Verification items for the finished model (mm, model axes). Face numbers are marked on the shaded views. A direction names the side the tool comes from. Give positions to 0.01 mm unless a question says otherwise; leave off trailing zeros. Loops run counter-clockwise (first coordinate to the right, second up) from the corner with the lowest first, then second, coordinate; pieces in that order, holes last. Notation, with made-up numbers: (16, 32.5) - (49, 32.5) arc R25 cw to (49, 70.5) - close; hole circle Ø1 at (44.5, 78.5). An arc over 180 degrees is marked (long way). Put each result on its own line as item: value. Start each with the question number.
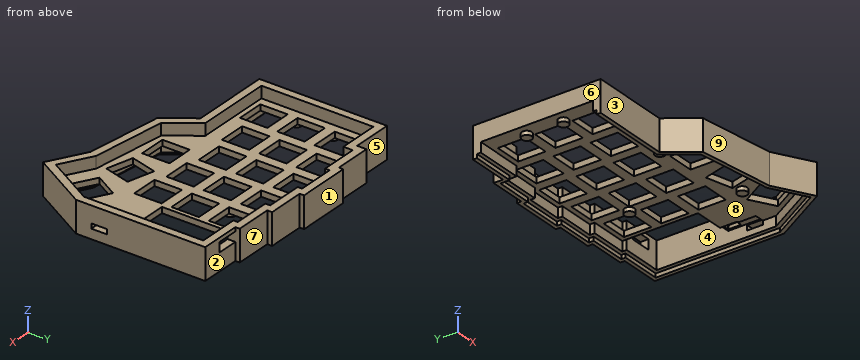
```python
from build123d import *

# Parameters (mm, degrees)
PAD005_DEPTH        = 16
POCKET_DEPTH        = 6
POCKET012_DEPTH     = 7
SKETCH001_W         = 14
SKETCH001_H         = 14
SKETCH001_W_2       = 20.75
SKETCH001_H_2       = 36.5
POCKET013_DEPTH     = 3
MIRROREDSKETCH009_R = 2.5
PAD_DEPTH           = 5
SKETCH_W            = 8
SKETCH_H            = 2.5
POCKET014_DEPTH     = 5
SKETCH015_W         = 11
SKETCH015_H         = 5
POCKET015_DEPTH     = 7
POCKET018_DEPTH     = 2
POCKET025_DEPTH     = 5
POCKET026_DEPTH     = 1.1


with BuildPart() as part:
    # MirroredSketch002 → Pad005 (new body)
    with BuildSketch(Plane.XY):
        Polygon((12.847899, 60.749919), (33.482443, 60.749919), (33.482443, 65.499919), (52.492443, 65.499919), (52.492443, 67.749919), (79.492443, 67.749919), (79.492443, 65.499919), (98.492443, 65.499919), (98.492443, 62.999919), (117.482443, 62.999919), (117.482443, 60.749919), (138.232443, 60.749919), (138.232443, -5.348885), (121.287497, -34.793261), (102.74032, -24.222717), (63.98748, -18.955575), (53.446293, -4.5), (12.847899, -4.5), align=None)
    extrude(amount=PAD005_DEPTH)

    # MirroredSketch005 → Pocket (cut)
    with BuildSketch(Plane.XY.offset(16)):
        Polygon((16.847899, -0.5), (16.847899, 56.75), (37.482443, 56.75), (37.482443, 61.499919), (56.492443, 61.499919), (56.492443, 63.749919), (75.492443, 63.749919), (75.492443, 61.499919), (94.492443, 61.499919), (94.492443, 58.999919), (113.482443, 58.999919), (113.482443, 56.749919), (134.232443, 56.749919), (134.232443, -4.280081), (119.807428, -29.345701), (104.047316, -20.363581), (66.215158, -15.221576), (55.48, -0.5), align=None)
    extrude(amount=-POCKET_DEPTH, mode=Mode.SUBTRACT)

    # MirroredSketch006 → Pocket012 (cut)
    with BuildSketch(Plane.XY):
        Polygon((-0.5, -0.5), (-0.5, 56.75), (37.482443, 56.75), (37.482443, 61.499919), (56.492443, 61.499919), (56.492443, 63.749919), (75.492443, 63.749919), (75.492443, 61.499919), (94.492443, 61.499919), (94.492443, 58.999919), (113.482443, 58.999919), (113.482443, 56.749919), (134.232443, 56.749919), (134.232443, -4.280081), (119.807428, -29.345701), (104.047316, -20.363581), (66.215158, -15.221576), (55.48, -0.5), align=None)
    extrude(amount=POCKET012_DEPTH, mode=Mode.SUBTRACT)

    # Sketch001 → Pocket013 (cut)
    with BuildSketch(Plane.XY.offset(10)):
        with Locations((75.62, -5.79)):
            Rectangle(SKETCH001_W, SKETCH001_H)
        Polygon((91.629303, 0.089303), (105.156052, -3.52), (101.546749, -17.046749), (88.02, -13.437445), align=None)
        Polygon((116.274632, -2.66), (128.398988, -9.66), (121.398988, -21.784355), (109.276749, -14.785577), align=None)
        with Locations((28.07, 47.16)):
            Rectangle(SKETCH001_W, SKETCH001_H)
        with Locations((28.07, 9.06)):
            Rectangle(SKETCH001_W, SKETCH001_H)
        with Locations((47.12, 51.97)):
            Rectangle(SKETCH001_W, SKETCH001_H)
        with Locations((47.12, 13.87)):
            Rectangle(SKETCH001_W, SKETCH001_H)
        with Locations((66.17, 54.27)):
            Rectangle(SKETCH001_W, SKETCH001_H)
        with Locations((66.17, 16.17)):
            Rectangle(SKETCH001_W, SKETCH001_H)
        with Locations((85.22, 51.87)):
            Rectangle(SKETCH001_W, SKETCH001_H)
        with Locations((85.22, 13.77)):
            Rectangle(SKETCH001_W, SKETCH001_H)
        with Locations((104.27, 49.54)):
            Rectangle(SKETCH001_W, SKETCH001_H)
        with Locations((47.12, 32.92)):
            Rectangle(SKETCH001_W, SKETCH001_H)
        with Locations((66.17, 35.22)):
            Rectangle(SKETCH001_W, SKETCH001_H)
        with Locations((28.07, 28.11)):
            Rectangle(SKETCH001_W, SKETCH001_H)
        with Locations((104.27, 30.49)):
            Rectangle(SKETCH001_W, SKETCH001_H)
        with Locations((104.27, 11.44)):
            Rectangle(SKETCH001_W, SKETCH001_H)
        with Locations((85.22, 32.82)):
            Rectangle(SKETCH001_W, SKETCH001_H)
        with Locations((123.857443, 38.499919)):
            Rectangle(SKETCH001_W_2, SKETCH001_H_2)
    extrude(amount=-POCKET013_DEPTH, mode=Mode.SUBTRACT)

    # MirroredSketch009 → Pad (join)
    with BuildSketch(Plane.XY.offset(10)):
        with Locations((18.61, 37.509997)):
            Circle(MIRROREDSKETCH009_R)
        with Locations((18.6, 18.76)):
            Circle(MIRROREDSKETCH009_R)
        with Locations((94.55, 41.252659)):
            Circle(MIRROREDSKETCH009_R)
        with Locations((61.84, 1.51)):
            Circle(MIRROREDSKETCH009_R)
        with Locations((108.3, -6.24)):
            Circle(MIRROREDSKETCH009_R)
    extrude(amount=-PAD_DEPTH)

    # Sketch → Pocket014 (cut)
    with BuildSketch(Plane.YZ.offset(138.3)):
        with Locations((6.479556, 6.26)):
            Rectangle(SKETCH_W, SKETCH_H)
    extrude(amount=-POCKET014_DEPTH, mode=Mode.SUBTRACT)

    # Sketch015 → Pocket015 (cut)
    with BuildSketch(Plane(origin=(6, 56.73, -16.55), x_dir=(1, 0, 0), z_dir=(0, -1, 0))):
        with Locations((116.982443, 28.05)):
            Rectangle(SKETCH015_W, SKETCH015_H)
    extrude(amount=-POCKET015_DEPTH, mode=Mode.SUBTRACT)

    # MirroredSketch013 → Pocket018 (cut)
    with BuildSketch(Plane.XY):
        Polygon((-2.5, 58.75), (35.482443, 58.75), (35.482443, 63.499919), (54.492443, 63.499919), (54.492443, 65.749919), (77.492443, 65.749919), (77.492443, 63.499919), (96.492443, 63.499919), (96.492443, 60.999919), (115.482443, 60.999919), (115.482443, 58.749919), (136.232443, 58.749919), (136.232443, -4.814483), (120.547462, -32.069481), (103.393818, -22.293149), (65.101319, -17.088576), (54.463147, -2.5), (-2.5, -2.5), align=None)
        Polygon((-0.5, -0.5), (-0.5, 56.75), (37.482443, 56.75), (37.482443, 61.499919), (56.492443, 61.499919), (56.492443, 63.749919), (75.492443, 63.749919), (75.492443, 61.499919), (94.492443, 61.499919), (94.492443, 58.999919), (113.482443, 58.999919), (113.482443, 56.749919), (134.232443, 56.749919), (134.232443, -4.280081), (119.807428, -29.345701), (104.047316, -20.363581), (66.215158, -15.221576), (55.48, -0.5), align=None, mode=Mode.SUBTRACT)
    extrude(amount=POCKET018_DEPTH, mode=Mode.SUBTRACT)

    # Sketch042 → Pocket025 (cut)
    with BuildSketch(Plane(origin=(131.5, 16.2, 8.1), x_dir=(1, 0, 0), z_dir=(0, 0, 1))):
        with BuildLine():
            ThreePointArc((-1.699662, -3.023679), (-1.602072, -3.215198), (-1.401398, -3.292227))
            Line((1.461956, -3.292227), (-1.401398, -3.292227))
            ThreePointArc((1.461956, -3.292227), (1.630798, -3.203454), (1.698398, -3.025076))
            Line((1.698398, 3.034671), (1.698398, -3.025076))
            ThreePointArc((1.698398, 3.034671), (1.611903, 3.194523), (1.444123, 3.264409))
            Line((-1.429415, 3.264409), (1.444123, 3.264409))
            ThreePointArc((-1.429415, 3.264409), (-1.620509, 3.185256), (-1.699662, 2.994162))
            Line((-1.699662, -3.023679), (-1.699662, 2.994162))
        make_face()
    extrude(amount=POCKET025_DEPTH, mode=Mode.SUBTRACT)

    # Sketch045 → Pocket026 (cut)
    with BuildSketch(Plane.XY.offset(7)):
        with BuildLine():
            Line((128.626114, 20.249919), (128.626114, 12.337918))
            ThreePointArc((128.626114, 12.337918), (128.679151, 12.055368), (128.83104, 11.811285))
            Line((128.83104, 11.811285), (129.270661, 11.331936))
            ThreePointArc((129.4413, 10.893416), (129.397137, 11.128691), (129.270661, 11.331936))
            Line((129.4413, 10.893416), (129.4413, 3.123712))
            ThreePointArc((129.4413, 3.123712), (129.629969, 2.668225), (130.085456, 2.479556))
            Line((130.085456, 2.479556), (134.232443, 2.479556))
            Line((134.232443, 20.249919), (134.232443, 2.479556))
            Line((128.626114, 20.249919), (134.232443, 20.249919))
        make_face()
    extrude(amount=POCKET026_DEPTH, mode=Mode.SUBTRACT)


solid = part.part
```
1) Section check B-B, the plane x = 84.5. Enter the section's corners in (y, z), plus the area to 3 significant figures.
2) Set-up check for the marked faces 1, 2, 3, 4 and 5: record each of +Z, -Z, +X, -X, +Y, -Y from which the full face is reachable in a straight line by a thin tool's end or side.
3) Section check A-A, the plane y = 30.5. State how many separate pieces and enclosed holes the cut face has, plus the area to 3 significant figures.
4) Draft check along Y on the marked faces 6, 7, 8 and 9. Enter one of: pulls with the +Y half, pulls with the -Y half, needs draft (parallel to the pull), parting line crosses it, or undercut.
5) Depth check by flat-ended pin: P1, Ø4, axis at x = 33.5, z = 12, coming from the +Y side; P2, Ø0.9, axis at y = -9, z = 8, coming from the -X side; P3, Ø2, axis at x = 23.5, z = 1, coming from the -Y side. Enter the tip coordinate at first touch or a pass-through.
6) Scan lines: line 1 along X through (y, z) = (42, 8.5); line 2 along X through (y, z) = (18.5, 11.5); line 3 along X through (y, z) = (59.5, 3). Record each from-to range of solid material in increasing order. Write a range as from..to.
7) Section check D-D, the plane x = 18.61. Enter the section's corners in (y, z), plus the area to 3 significant figures.
Results are:
1. outline: (-21.74, 0) - (-19.73, 0) - (-19.73, 2) - (-17.71, 2) - (-17.71, 7) - (6.77, 7) - (6.77, 10) - (-17.71, 10) - (-17.71, 16) - (-21.74, 16) - close; (20.77, 7) - (25.82, 7) - (25.82, 10) - (20.77, 10) - close; (39.82, 7) - (44.87, 7) - (44.87, 10) - (39.82, 10) - close; (58.87, 7) - (61.5, 7) - (61.5, 2) - (63.5, 2) - (63.5, 0) - (65.5, 0) - (65.5, 16) - (61.5, 16) - (61.5, 10) - (58.87, 10) - close
1. area: 232 mm2
2. face 1: +Z, -Z, +X, -X, +Y
2. face 2: +Z, -Z, +X, +Y
2. face 3: +Z, -Z, -X, -Y
2. face 4: none
2. face 5: +Z, -Z, -X, +Y
3. separate pieces: 7
3. enclosed holes: 0
3. area: 176 mm2
4. face 6: needs draft
4. face 7: pulls with the +Y half
4. face 8: undercut
4. face 9: pulls with the -Y half
5. P1: stops at y = 65.5
5. P2: stops at x = 56.4
5. P3: stops at y = -4.5
6. line 1: x = 12.85..21.07, 35.07..59.17, 73.17..113.48, 134.23..138.23
6. line 2: x = 12.85..16.85, 134.23..138.23
6. line 3: x = 12.85..37.48, 94.49..138.23
7. outline: (-4.5, 0) - (-2.5, 0) - (-2.5, 2) - (-0.5, 2) - (-0.5, 7) - (16.26, 7) - (16.26, 5) - (21.26, 5) - (21.26, 7) - (35.01, 7) - (35.01, 5) - (40.01, 5) - (40.01, 7) - (56.75, 7) - (56.75, 2) - (58.75, 2) - (58.75, 0) - (60.75, 0) - (60.75, 16) - (56.75, 16) - (56.75, 10) - (-0.5, 10) - (-0.5, 16) - (-4.5, 16) - close
7. area: 312 mm2
